```python
from build123d import *

# Parameters (mm, degrees)
SKETCH1_W                        = 42
SKETCH1_H                        = 70
BOSS_EXTRUDE1_DEPTH              = 6
SKETCH2_W                        = 5
SKETCH2_H                        = 6
CUT_EXTRUDE1_DEPTH               = 9
F_12_0MM_DOWEL_HOLE1_D           = 12
F_12_0MM_DOWEL_HOLE1_DEPTH       = 50
F_12_0MM_DOWEL_HOLE1_CSINK_D     = 12.05
F_12_0MM_DOWEL_HOLE1_CSINK_ANGLE = 90
F_12_0MM_DOWEL_HOLE1_TIP         = 3.605163714


with BuildPart() as part:
    # Sketch1 → Boss-Extrude1 (new body)
    with BuildSketch(Plane.XY):
        with Locations((-9.849777317, 69.889242879)):
            Rectangle(SKETCH1_W, SKETCH1_H)
    extrude(amount=BOSS_EXTRUDE1_DEPTH)

    # Sketch2 → Cut-Extrude1 (cut)
    with BuildSketch(Plane.XY):
        with Locations((-4.211301735, 38.120527714)):
            Rectangle(SKETCH2_W, SKETCH2_H)
        with Locations((-15.91362892, 38.2243844)):
            Rectangle(SKETCH2_W, SKETCH2_H)
    extrude(amount=CUT_EXTRUDE1_DEPTH, mode=Mode.SUBTRACT)

    # Ø12.0mm Dowel Hole1
    with Locations(Plane(origin=(0, 0, 0), x_dir=(-1, 0, 0), z_dir=(0, 0, -1))):
        with Locations((10.096577426, 49.898434055)):
            CounterSinkHole(F_12_0MM_DOWEL_HOLE1_D / 2, F_12_0MM_DOWEL_HOLE1_CSINK_D / 2, depth=F_12_0MM_DOWEL_HOLE1_DEPTH, counter_sink_angle=F_12_0MM_DOWEL_HOLE1_CSINK_ANGLE)
            with Locations((0, 0, -(F_12_0MM_DOWEL_HOLE1_DEPTH + F_12_0MM_DOWEL_HOLE1_TIP / 2))):  # 118° drill point
                Cone(0, F_12_0MM_DOWEL_HOLE1_D / 2, F_12_0MM_DOWEL_HOLE1_TIP, mode=Mode.SUBTRACT)


solid = part.part
```
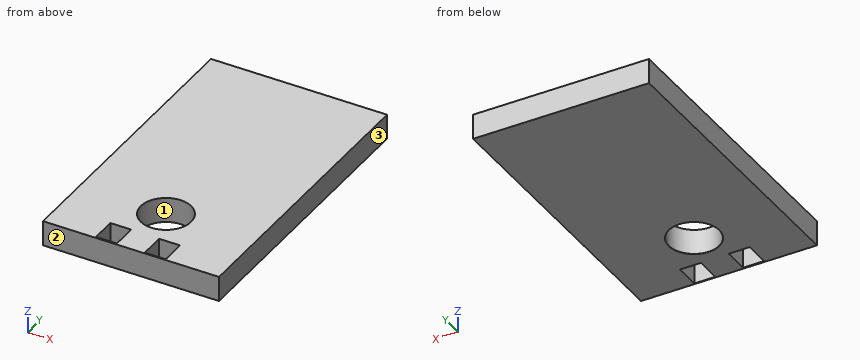
Part model, mm, in its own coordinate system. Face numbers are marked on the shaded views. Coordinates: 2 decimals unless noted, no trailing zeros. Write each loop counter-clockwise with the first axis right and the second up, starting at its lowest first coordinate (ties: lowest second). Pieces come first, ordered by that corner, then holes.
Item 1: Mould opens along X. For the marked faces 1, 2 and 3 say: released by +X, released by -X, zero draft, split by the parting line, or undercut.
Item 2: Pin check, flat tip, straight feed: pin 1 (11 mm diameter, centred on x = -10.1, y = 49.9, fed in from -Z). Stop position of the tip, or through.
Item 3: Slice it at B-B (y = 39). Write the cut outline in (x, z), and give its area (3 significant figures).
Item 4: Probe line 1 (X direction, y = 50, z = 0.55); line 2 (X direction, y = 40, z = 4.45); line 3 (Y direction, x = -10.5, z = 5.45). List the from-to ranges inside material, lowest first.
Item 5: Slice it at C-C (z = 3.8). Write the cut outline in (x, y), and give its area (3 significant figures).
Item 6: Slice it at A-A (x = -17.5). Write the cut outline in (y, z).
Results found:
1. face 1: undercut
1. face 2: zero draft
1. face 3: released by +X
2. pin 1: passes through
3. outline: (-30.85, 0) - (-18.41, 0) - (-18.41, 6) - (-30.85, 6) - close; (-13.41, 0) - (-6.71, 0) - (-6.71, 6) - (-13.41, 6) - close; (-1.71, 0) - (11.15, 0) - (11.15, 6) - (-1.71, 6) - close
3. area: 192 mm2
4. line 1: x = -30.85 to -16.1, -4.1 to 11.15
4. line 2: x = -30.85 to -18.41, -13.41 to -6.71, -1.71 to 11.15
4. line 3: y = 34.89 to 43.91, 55.88 to 104.89
5. outline: (-30.85, 34.89) - (11.15, 34.89) - (11.15, 104.89) - (-30.85, 104.89) - close; hole (-18.41, 35.22) - (-13.41, 35.22) - (-13.41, 41.22) - (-18.41, 41.22) - close; hole circle Ø12 at (-10.1, 49.9); hole (-6.71, 35.12) - (-1.71, 35.12) - (-1.71, 41.12) - (-6.71, 41.12) - close
5. area: 2,770 mm2
6. outline: (34.89, 0) - (35.22, 0) - (35.22, 6) - (34.89, 6) - close; (41.22, 0) - (104.89, 0) - (104.89, 6) - (41.22, 6) - close
